Here's how the part is built. I have some questions about the finished solid (model axes, mm). Round coordinates to 2 decimals unless told otherwise and drop trailing zeros. Loops run counter-clockwise (first coordinate to the right, second up) from the corner with the lowest first, then second, coordinate; pieces in that order, holes last. Notation, with made-up numbers: M 9.25,-35.75 L 59.25,-35.75 A23 ccw 59.25,-18.75 Z; hole C 55.25,-14.5 d2. An arc over 180 degrees is marked long. Use a Markdown table: item, result.
```python
from build123d import *

# Parameters (mm, degrees)
F1_DEPTH    = 2.032
F2_T2_ANGLE = 50.6284103455
F2_T4_ANGLE = 50.6284103455
F2_T6_ANGLE = 50.6284103455
F2_T8_ANGLE = 50.6284103455
F3_T1_DEPTH = 26.2461176682
F3_T3_DEPTH = 24.8658132399
F3_T5_DEPTH = 24.86581324
F3_T7_DEPTH = 26.2461176682
F3_T9_DEPTH = 8.2601420581


# Not quite as in the source:
# - a fillet or chamfer that OpenCascade refuses, or shapes differently, is made with other operations: its cross-section is extruded or revolved along the edge and cut away or added


with BuildPart() as f1:
    # F0 (on Top) → F1 (new body)
    with BuildSketch(Plane.XY):
        with BuildLine():
            Line((-4.1300710291, 54.8246689141), (-24.0261886972, 54.8246689141))
            ThreePointArc((-24.0261886972, 54.8246689141), (-18.5763848247, 37.4605098755), (-16.7346344691, 19.3546451628))
            ThreePointArc((-16.7346344691, 19.3546451628), (-18.5763848247, 1.2487804501), (-24.0261886972, -16.1153785884))
            Line((-24.0261886972, -16.1153785884), (-4.1300710291, -16.1153785884))
            Line((-4.1300710291, -16.1153785884), (-4.1300710291, 11.5803927183))
            Line((-4.1300710291, 11.5803927183), (4.1300710291, 11.5803927183))
            Line((4.1300710291, 11.5803927183), (4.1300710291, -16.1153785884))
            Line((4.1300710291, -16.1153785884), (24.0261886972, -16.1153785884))
            ThreePointArc((24.0261886972, -16.1153785884), (18.5763848247, 1.2487804501), (16.7346344691, 19.3546451628))
            ThreePointArc((16.7346344691, 19.3546451628), (18.5763848247, 37.4605098755), (24.0261886972, 54.8246689141))
            Line((24.0261886972, 54.8246689141), (4.1300710291, 54.8246689141))
            Line((4.1300710291, 54.8246689141), (4.1300710291, 27.1288976073))
            Line((4.1300710291, 27.1288976073), (-4.1300710291, 27.1288976073))
            Line((-4.1300710291, 27.1288976073), (-4.1300710291, 54.8246689141))
        make_face()
    extrude(amount=F1_DEPTH)

    # F2: chamfer of 1.27 on 4 edges, made by hand

    # F2_s1 → F2_t2 (revolve, cut)
    with BuildSketch(Plane(origin=(26.9800180079, 57.0400631379, 0), x_dir=(0, 0, 1), z_dir=(0.4275819968, 0.9039765683, 0))):
        Polygon((2.032, -3.0522508854), (0.762, -1.7822508854), (2.032, -1.7822508854), align=None)
    revolve(axis=Axis((106.6530048847, 19.3546451628, 2.032), (0, 0, 1)), revolution_arc=F2_T2_ANGLE, mode=Mode.SUBTRACT)

    # F2_s3 → F2_t4 (revolve, cut)
    with BuildSketch(Plane(origin=(12.017944167, -25.4078516136, 0), x_dir=(0, 0, 1), z_dir=(0.4275819968, -0.9039765683, 0))):
        Polygon((0, -13.499144765), (1.27, -14.769144765), (0, -14.769144765), align=None)
    revolve(axis=Axis((106.6530048847, 19.3546451628, 0), (0, 0, -1)), revolution_arc=F2_T4_ANGLE, mode=Mode.SUBTRACT)

    # F2_s5 → F2_t6 (revolve, cut)
    with BuildSketch(Plane(origin=(-12.017944167, -25.4078516136, 0), x_dir=(0, 0, 1), z_dir=(-0.4275819968, -0.9039765683, 0))):
        Polygon((2.032, 13.499144765), (0.762, 14.769144765), (2.032, 14.769144765), align=None)
    revolve(axis=Axis((-106.6530048847, 19.3546451628, 2.032), (0, 0, 1)), revolution_arc=F2_T6_ANGLE, mode=Mode.SUBTRACT)

    # F2_s7 → F2_t8 (revolve, cut)
    with BuildSketch(Plane(origin=(-26.9800180079, 57.0400631379, 0), x_dir=(0, 0, 1), z_dir=(-0.4275819968, 0.9039765683, 0))):
        Polygon((1.27, 1.7822508854), (0, 3.0522508854), (0, 1.7822508854), align=None)
    revolve(axis=Axis((-106.6530048847, 19.3546451628, 0), (0, 0, -1)), revolution_arc=F2_T8_ANGLE, mode=Mode.SUBTRACT)

    # F3: fillet of radius 1.27 on 12 edges, made by hand

    # F3_s2 → F3_t1 (cut)
    with BuildSketch(Plane.YZ.offset(-27.2011886972)):
        with BuildLine():
            ThreePointArc((54.8246689141, 1.27), (54.4526945262, 0.3719743879), (53.5546689141, 0))
            Line((53.5546689141, 0), (54.8246689141, 0))
            Line((54.8246689141, 0), (54.8246689141, 1.27))
        make_face()
        with BuildLine():
            ThreePointArc((-16.1153785884, 1.27), (-15.7434042005, 0.3719743879), (-14.8453785884, 0))
            Line((-14.8453785884, 0), (-16.1153785884, 0))
            Line((-16.1153785884, 0), (-16.1153785884, 1.27))
        make_face()
    extrude(amount=F3_T1_DEPTH, mode=Mode.SUBTRACT)

    # F3_s4 → F3_t3 (cut)
    with BuildSketch(Plane.YZ.offset(-25.820884269)):
        with BuildLine():
            ThreePointArc((54.8246689141, 0.762), (54.4526945262, 1.6600256121), (53.5546689141, 2.032))
            Line((53.5546689141, 2.032), (54.8246689141, 2.032))
            Line((54.8246689141, 2.032), (54.8246689141, 0.762))
        make_face()
        with BuildLine():
            ThreePointArc((-16.1153785884, 0.762), (-15.7434042005, 1.6600256121), (-14.8453785884, 2.032))
            Line((-14.8453785884, 2.032), (-16.1153785884, 2.032))
            Line((-16.1153785884, 2.032), (-16.1153785884, 0.762))
        make_face()
    extrude(amount=F3_T3_DEPTH, mode=Mode.SUBTRACT)

    # F3_s6 → F3_t5 (cut)
    with BuildSketch(Plane.YZ.offset(0.9550710291)):
        with BuildLine():
            ThreePointArc((54.8246689141, 0.762), (54.4526945262, 1.6600256121), (53.5546689141, 2.032))
            Line((53.5546689141, 2.032), (54.8246689141, 2.032))
            Line((54.8246689141, 2.032), (54.8246689141, 0.762))
        make_face()
        with BuildLine():
            ThreePointArc((-16.1153785884, 0.762), (-15.7434042005, 1.6600256121), (-14.8453785884, 2.032))
            Line((-14.8453785884, 2.032), (-16.1153785884, 2.032))
            Line((-16.1153785884, 2.032), (-16.1153785884, 0.762))
        make_face()
    extrude(amount=F3_T5_DEPTH, mode=Mode.SUBTRACT)

    # F3_s8 → F3_t7 (cut)
    with BuildSketch(Plane.YZ.offset(0.9550710291)):
        with BuildLine():
            ThreePointArc((54.8246689141, 1.27), (54.4526945262, 0.3719743879), (53.5546689141, 0))
            Line((53.5546689141, 0), (54.8246689141, 0))
            Line((54.8246689141, 0), (54.8246689141, 1.27))
        make_face()
        with BuildLine():
            ThreePointArc((-16.1153785884, 1.27), (-15.7434042005, 0.3719743879), (-14.8453785884, 0))
            Line((-14.8453785884, 0), (-16.1153785884, 0))
            Line((-16.1153785884, 0), (-16.1153785884, 1.27))
        make_face()
    extrude(amount=F3_T7_DEPTH, mode=Mode.SUBTRACT)

    # F3_s10 → F3_t9 (cut)
    with BuildSketch(Plane.YZ.offset(-4.1300710291)):
        with BuildLine():
            ThreePointArc((11.5803927183, 0.762), (11.9523671062, 1.6600256121), (12.8503927183, 2.032))
            Line((12.8503927183, 2.032), (11.5803927183, 2.032))
            Line((11.5803927183, 2.032), (11.5803927183, 0.762))
        make_face()
        with BuildLine():
            ThreePointArc((11.5803927183, 1.27), (11.9523671062, 0.3719743879), (12.8503927183, 0))
            Line((12.8503927183, 0), (11.5803927183, 0))
            Line((11.5803927183, 0), (11.5803927183, 1.27))
        make_face()
        with BuildLine():
            ThreePointArc((27.1288976073, 1.27), (26.7569232194, 0.3719743879), (25.8588976073, 0))
            Line((25.8588976073, 0), (27.1288976073, 0))
            Line((27.1288976073, 0), (27.1288976073, 1.27))
        make_face()
        with BuildLine():
            ThreePointArc((27.1288976073, 0.762), (26.7569232194, 1.6600256121), (25.8588976073, 2.032))
            Line((25.8588976073, 2.032), (27.1288976073, 2.032))
            Line((27.1288976073, 2.032), (27.1288976073, 0.762))
        make_face()
    extrude(amount=F3_T9_DEPTH, mode=Mode.SUBTRACT)


solid = f1.part
```
Q1. Imagine slicing it at A-A, the plane z = 1.45. Please give me the cut outline in (x, y), then the cut area to 3 significant figures.
Return value:
| item | result |
|---|---|
| outline | M -23.19,-15.91 L -4.13,-15.91 L -4.13,11.78 L 4.13,11.78 L 4.13,-15.91 L 23.19,-15.91 A90.61 cw 23.19,54.62 L 4.13,54.62 L 4.13,26.93 L -4.13,26.93 L -4.13,54.62 L -23.19,54.62 A90.61 cw Z |
| area | 2,140 mm^2 |
Q2. We'd pull the mould along Y, two halves only. Please class faces 1 (the conical face through (16.3, 19.9, 1.2)), 2 (the flat face through (4.13, -1, 1)), 3 (the conical face through (-16.3, 18.8, 1.2)): pulls with the +Y half, pulls with the -Y half, needs draft (parallel to the pull), parting line crosses it, or undercut.
Return value:
| item | result |
|---|---|
| face 1 | undercut |
| face 2 | needs draft |
| face 3 | undercut |
Q3. I need wall thicknesses on line 1 (X direction, y = 47, z = 0.4); line 2 (X direction, y = -5.5, z = 0.3); line 3 (Y direction, x = 11, z = 1.5). Which ranges of each line are inside material? Lowest first, please. Write a range as from..to.
Return value:
| item | result |
|---|---|
| line 1 | x = -20.18..-4.13, 4.13..20.18 |
| line 2 | x = -19.23..-4.13, 4.13..19.23 |
| line 3 | y = -15.88..54.59 |
Q4. Will these pins go through, and if not, where does the flat tip stop? P1, Ø0.6, axis at y = 0.5, z = 1.5, coming from the +X side; P2, Ø3, axis at x = 1.5, y = 6, coming from the -Z side.
Return value:
| item | result |
|---|---|
| P1 | stops at x = 18.29 |
| P2 | passes through |
